Job drawing, mm, ordinate dimensions from the low corner. One solid piece. Round coordinates to 2 decimals unless told otherwise and drop trailing zeros. Loops run counter-clockwise (first coordinate to the right, second up) from the corner with the lowest first, then second, coordinate; pieces in that order, holes last. Notation, with made-up numbers: M 46.5,75 L 55.5,75 A5 ccw 55.5,79 Z; hole C 37,30 d11. An arc over 180 degrees is marked long. Use a Markdown table: item, result. Add a question column.
(1) Wall check: L1, parallel to X at y = 76.2, z = 2.25; L2, parallel to Y at x = 250, z = 1.5 (1 decimal); L3, parallel to X at y = 287.5, z = 5.5 (1 decimal). Give the ranges that are in metal, low to high.
(2) Band-saw the part on D-D, the plane x = 333.5. Write the cut outline in (y, z) (1 decimal).
(3) Band-saw the part on C-C, the plane y = 342.9. Write the cut outline in (x, z) (1 decimal), and give its area (3 significant figures).
(4) Band-saw the part on B-B, the plane x = 190.5. Write the cut outline in (y, z) (1 decimal), and give its area (3 significant figures).
(5) Band-saw the part on A-A, the plane z = 7.5. Give the number of separate pieces and of enclosed holes in the cut face, and give its area (3 significant figures).
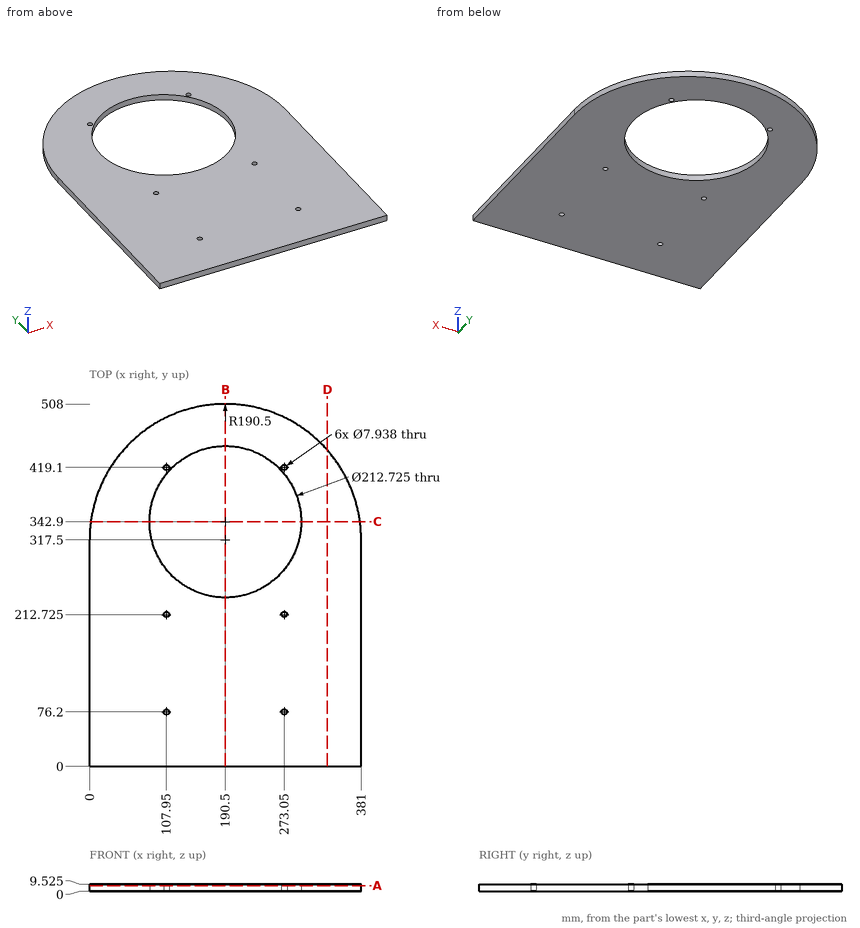
Return value:
| question | item | result |
|---|---|---|
| 1 | L1 | 0 to 103.98, 111.92 to 269.08, 277.02 to 381 |
| 1 | L2 | 0 to 254.7, 431.1 to 498.5 |
| 1 | L3 | 0 to 99.7, 281.3 to 381 |
| 2 | outline | M 0,0 L 443.4,0 L 443.4,9.5 L 0,9.5 Z |
| 3 | outline | M 1.7,0 L 84.1,0 L 84.1,9.5 L 1.7,9.5 Z; M 296.9,0 L 379.3,0 L 379.3,9.5 L 296.9,9.5 Z |
| 3 | area | 1,570 mm^2 |
| 4 | outline | M 0,0 L 236.5,0 L 236.5,9.5 L 0,9.5 Z; M 449.3,0 L 508,0 L 508,9.5 L 449.3,9.5 Z |
| 4 | area | 2,810 mm^2 |
| 5 | separate pieces | 1 |
| 5 | enclosed holes | 7 |
| 5 | area | 142,000 mm^2 |
